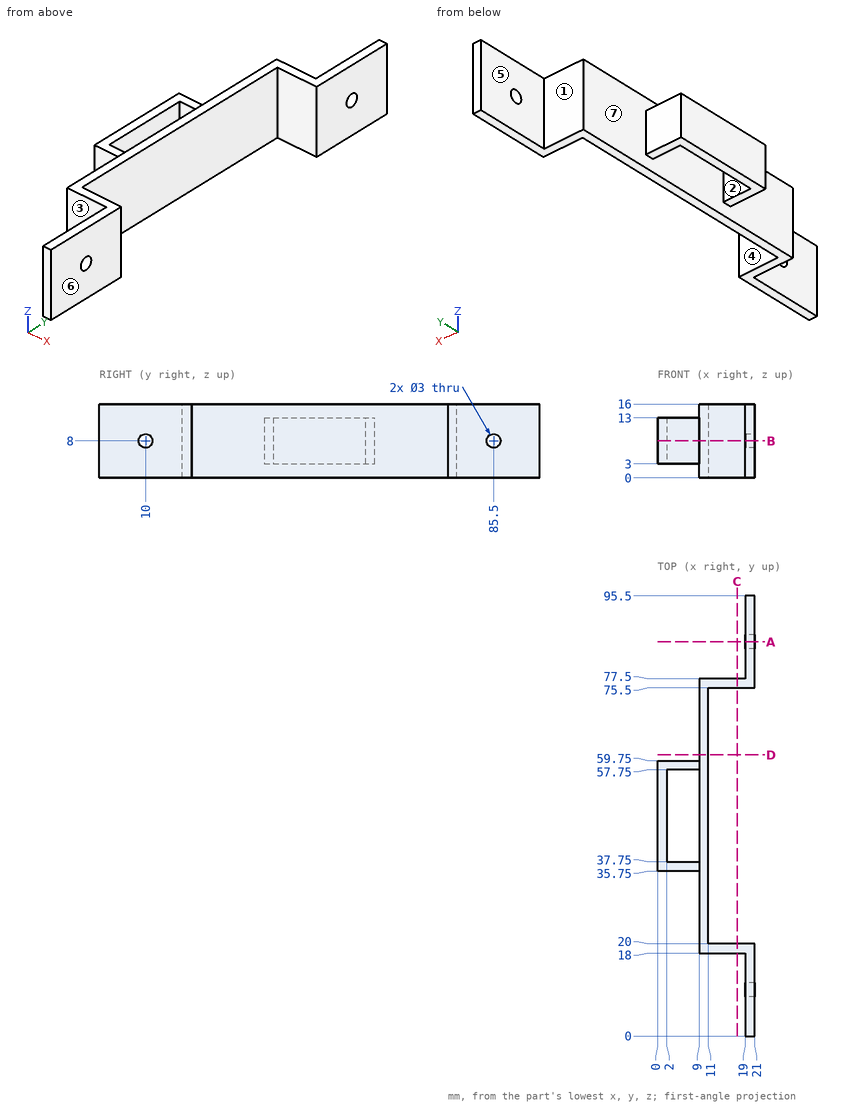
Here's the drawing with two shaded views (mm, measured from the low corner). I have some questions. A direction names the side the tool comes from. Give positions to 0.01 mm unless a question says otherwise; leave off trailing zeros. Write each loop counter-clockwise with the first axis right and the second up, starting at its lowest first coordinate (ties: lowest second). Pieces come first, ordered by that corner, then holes. Notation, with made-up numbers: (49, 68) -> (93, 68) arc R17 ccw to (93, 77) -> close; hole circle Ø5 at (-37, 62.5). An arc over 180 degrees is marked (long way). Answer as a JSON object with one key per item and string values. Group by question number.
Item 1: Suppose I cut it at C-C (x = 17.25). Please give me the cut outline in (y, z).
Item 2: For the marked faces 1, 2, 3 and 4, which set-ups out of +Z, -Z, +X, -X, +Y, -Y let a thin tool reach every point of the face, with its end or its side?
Item 3: Suppose I cut it at D-D (y = 61). Please give me the cut outline in (x, z).
Item 4: Please list where these lines run through material, in increasing order: line 1 (Y direction, x = 20.4, z = 8); line 2 (Y direction, x = 16.25, z = 6); line 3 (Z direction, x = 20.35, y = 85.5). Write a range as [from, to].
Item 5: We'd pull the mould along X, two halves only. Please class the marked faces 5, 6 and 7: +X half, -X half, draft (parallel to the pull), parting line (faces both ways), or undercut.
Item 6: Suppose I cut it at A-A (y = 85.5). Please give me the cut outline in (x, z), plus the area to 3 significant figures.
Item 7: I'm going to push flat-ended pins straight in: P1, Ø2.5, axis at x = 5.5, z = 8, coming from the -Y side; P2, Ø7.5, axis at x = 4.5, z = 9.5, coming from the +Y side; P3, Ø2.5, axis at y = 10, z = 8, coming from the +X side (3 decimals); P4, Ø1, axis at y = 36.5, z = 8.5, coming from the +X side. Where does each tip first touch, or does it pass through?
Item 8: Suppose I cut it at B-B (z = 8). Please give me the cut outline in (x, y).
Findings:
{
 "1": {"outline": "(18, 0) -> (20, 0) -> (20, 16) -> (18, 16) -> close; (75.5, 0) -> (77.5, 0) -> (77.5, 16) -> (75.5, 16) -> close"},
 "2": {"face 1": "+Z, -Z, -X, +Y", "face 2": "+Z, -Z", "face 3": "+Z, -Z, -X, -Y", "face 4": "+Z, -Z, +X"},
 "3": {"outline": "(9, 0) -> (11, 0) -> (11, 16) -> (9, 16) -> close"},
 "4": {"line 1": "y = [0, 8.5], [11.5, 20], [75.5, 84], [87, 95.5]", "line 2": "y = [18, 20], [75.5, 77.5]", "line 3": "z = [0, 6.5], [9.5, 16]"},
 "5": {"face 5": "-X half", "face 6": "+X half", "face 7": "undercut"},
 "6": {"outline": "(19, 0) -> (21, 0) -> (21, 6.5) -> (19, 6.5) -> close; (19, 9.5) -> (21, 9.5) -> (21, 16) -> (19, 16) -> close", "area": "26.0 mm²"},
 "7": {"P1": "stops at y = 35.75", "P2": "stops at y = 59.75", "P3": "passes through", "P4": "stops at x = 11"},
 "8": {"outline": "(0, 35.75) -> (9, 35.75) -> (9, 18) -> (19, 18) -> (19, 11.5) -> (21, 11.5) -> (21, 20) -> (11, 20) -> (11, 75.5) -> (21, 75.5) -> (21, 84) -> (19, 84) -> (19, 77.5) -> (9, 77.5) -> (9, 59.75) -> (0, 59.75) -> close; (19, 0) -> (21, 0) -> (21, 8.5) -> (19, 8.5) -> close; (19, 87) -> (21, 87) -> (21, 95.5) -> (19, 95.5) -> close; hole (2, 37.75) -> (9, 37.75) -> (9, 57.75) -> (2, 57.75) -> close"}
}
